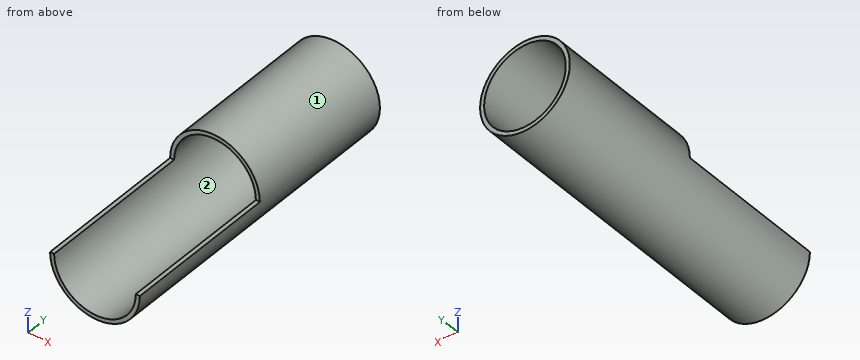
```python
from build123d import *

# Parameters (mm, degrees)
F0_R     = 44.45
F1_DEPTH = 300
F3_DEPTH = 150
F5_D     = 80.9
F5_DEPTH = 300


with BuildPart() as f1:
    # F0 (on Front) → F1 (new body)
    with BuildSketch(Plane.XZ):
        Circle(F0_R)
    extrude(amount=F1_DEPTH)

    # F2 (on face) → F3 (cut)
    with BuildSketch(Plane.XZ.offset(300)):
        with BuildLine():
            ThreePointArc((44.45, 0), (0, 44.45), (-44.45, 0))
            Line((-44.45, 0), (44.45, 0))
        make_face()
    extrude(amount=-F3_DEPTH, mode=Mode.SUBTRACT)

    # F5
    with Locations(Plane(origin=(0, 0, 0), x_dir=(-1, 0, 0), z_dir=(0, 1, 0))):
        with Locations((0, 0)):
            Hole(F5_D / 2, depth=F5_DEPTH)


solid = f1.part
```
For this review, take the finished solid that the model builds, in its own axes (mm). Face numbers are marked on the shaded views. Round coordinates to 2 decimals unless told otherwise and drop trailing zeros. Write each loop counter-clockwise with the first axis right and the second up, starting at its lowest first coordinate (ties: lowest second). Pieces come first, ordered by that corner, then holes. Notation, with made-up numbers: (85.25, -15) - (98.25, -15) arc R32 cw to (98.25, 14) - close; hole circle Ø6 at (60, 19). An arc over 180 degrees is marked (long way). Put each result on its own line as item: value.
Q1. We need section B-B (z = -12). Give the boundary of the cut face in (x, y), and give its area (3 significant figures).
Solved:
outline: (-42.8, -300) - (-38.63, -300) - (-38.63, 0) - (-42.8, 0) - close; (38.63, -300) - (42.8, -300) - (42.8, 0) - (38.63, 0) - close
area: 2,500 mm2
Q2. We need section C-C (y = -70). Give the boundary of the cut face in (x, z).
Solved:
outline: circle Ø88.9 at (0, 0); hole circle Ø80.9 at (0, 0)
Q3. We need section A-A (x = 0). Give the boundary of the cut face in (y, z), and give its area (3 significant figures).
Solved:
outline: (-300, -44.45) - (0, -44.45) - (0, -40.45) - (-300, -40.45) - close; (-150, 40.45) - (0, 40.45) - (0, 44.45) - (-150, 44.45) - close
area: 1,800 mm2
Q4. Mouldability with a two-part tool opening along Z and no side actions: class the marked faces 1 and 2 as released by +Z, released by -Z, zero draft, split by the parting line, or undercut.
Solved:
face 1: split by the parting line
face 2: undercut
Q5. We need section D-D (y = -218). Give the boundary of the cut face in (x, z), and give its area (3 significant figures).
Solved:
outline: (-44.45, 0) arc R44.45 ccw to (44.45, 0) - (40.45, 0) arc R40.45 cw to (-40.45, 0) - close
area: 533 mm2
Q6. Insertion check: pin 1 Ø1 at (y, z) = (-246.5, -22) entering from -X; pin 2 Ø1.2 at (x, y) = (43.5, -224) entering from +Z; pin 3 Ø13.5 at (x, z) = (-13, 26.5) entering from -Y; pin 4 Ø5 at (y, z) = (-150, -30.5) entering from -X. Each pin has a flat end and moves straight along its axis. Give the tip position at first contact, or say it passes through.
Solved:
pin 1: stops at x = -38.9
pin 2: stops at z = 0
pin 3: passes through
pin 4: stops at x = -34.52
Q7. Wall thickness on probe 1 along X at (y, z) = (-134, 0); probe 2 along X at (y, z) = (-94, -22.5): over which ranges is each line inside the solid? List them lowest first.
Solved:
probe 1: x = -44.45 to -40.45, 40.45 to 44.45
probe 2: x = -38.33 to -33.61, 33.61 to 38.33
